Autodesk Inventor part; units mm, degrees
ref_plane "YZ Plane" through (0, 0, 0) normal (1, 0, 0) x (0, 1, 0)
ref_plane "XZ Plane" through (0, 0, 0) normal (0, 1, 0) x (-1, 0, 0)
ref_plane "XY Plane" through (0, 0, 0) normal (0, 0, 1) x (1, 0, 0)
sketch "Sketch1" plane through (0, 0, 0) normal (0, 0, 1) x (1, 0, 0)
  line L0 (-35.3228, 16.049) -> (-9.9228, 16.049)
  line L1 (-9.9228, 16.049) -> (-9.9228, -34.751)
  line L2 (-9.9228, -34.751) -> (-35.3228, -34.751)
  line L3 (-35.3228, -34.751) -> (-35.3228, 16.049)
  line L4 (-13.0978, 12.874) -> (-32.1478, 12.874)
  line L5 (-32.1478, 12.874) -> (-32.1478, -31.576)
  line L6 (-32.1478, -31.576) -> (-13.0978, -31.576)
  line L7 (-13.0978, -31.576) -> (-13.0978, 12.874)
  point P0 (0, 0)
  dimension "d0" = 25.4
  dimension "d1" = 50.8
  dimension "d2" = 3.175
extrude "Extrusion1" add sketch "Sketch1" along normal blind 977.9
sketch "Sketch2" plane through (-35.3228, -34.751, 0) normal (-1, 0, 0) x (0, 0, 1)
  line L0 (0, 0) -> (0, 50.8) construction
  line L1 (0, 25.4) -> (25.4, 25.4) construction
  circle A0 centre (25.4, 25.4) radius 12.7
  point P0 (0, 34.751)
  dimension "d5" = 25.4
  dimension "d9" = 25.4
extrude "Extrusion2" cut sketch "Sketch2" against normal blind 12.7
sketch "Sketch3" plane through (-35.3228, -34.751, 0) normal (-1, 0, 0) x (0, 0, 1)
  line L0 (977.9, 50.8) -> (977.9, 0) construction
  line L1 (977.9, 25.4) -> (800.1, 25.4) construction
  circle A0 centre (800.1, 25.4) radius 14.2875
  point P0 (0, 34.751)
  dimension "d10" = 177.8
  dimension "d11" = 28.575
extrude "Extrusion3" cut sketch "Sketch3" against normal blind 25.4
sketch "Sketch4" plane through (-35.3228, -34.751, 0) normal (-1, 0, 0) x (0, 0, 1)
  line L0 (977.9, 50.8) -> (977.9, 0) construction
  line L1 (977.9, 25.4) -> (419.1, 25.4) construction
  circle A0 centre (419.1, 25.4) radius 14.2875
  point P0 (0, 34.751)
  dimension "d14" = 558.8
  dimension "d15" = 28.575
extrude "Extrusion4" cut sketch "Sketch4" against normal blind 25.4
sketch "Sketch5" plane through (-35.3228, -34.751, 0) normal (-1, 0, 0) x (0, 0, 1)
  circle A0 centre (419.1, 25.4) radius 14.2875 construction
  line L0 (419.1, 25.4) -> (401.1395, 7.4395) construction
  line L1 (419.1, 25.4) -> (444.5, 25.4) construction
  line L2 (419.1, 25.4) -> (437.0605, 43.3605) construction
  circle A1 centre (401.1395, 7.4395) radius 2.032
  circle A2 centre (437.0605, 43.3605) radius 2.032
  point P0 (0, 34.751)
  dimension "d18" = 25.4
  dimension "d19" = 135
  dimension "d20" = 25.4
  dimension "d21" = 4.064
  dimension "d22" = 4.064
extrude "Extrusion5" cut sketch "Sketch5" against normal blind 25.4
sketch "Sketch7" plane through (-9.9228, -34.751, 0) normal (1, 0, 0) x (0, 0, -1)
  line L0 (0, 0) -> (0, 50.8) construction
  line L1 (0, 25.4) -> (-25.4, 25.4) construction
  circle A0 centre (-25.4, 25.4) radius 14.2875
  point P0 (0, 34.751)
  dimension "d34" = 25.4
  dimension "d35" = 28.575
extrude "Extrusion7" cut sketch "Sketch7" against normal blind 12.7
sketch "Sketch8" plane through (-9.9228, -34.751, 0) normal (1, 0, 0) x (0, 0, -1)
  circle A0 centre (-25.4, 25.4) radius 14.2875 construction
  line L0 (-25.4, 25.4) -> (-25.4, 49.2125) construction
  line L1 (-25.4, 49.2125) -> (-4.7778, 37.3063) construction
  line L2 (-4.7778, 37.3063) -> (-4.7778, 13.4938) construction
  line L3 (-4.7778, 13.4938) -> (-25.4, 1.5875) construction
  line L4 (-25.4, 1.5875) -> (-46.0222, 13.4937) construction
  line L5 (-46.0222, 13.4937) -> (-46.0222, 37.3062) construction
  line L6 (-46.0222, 37.3062) -> (-25.4, 49.2125) construction
  circle A1 centre (-4.7778, 37.3063) radius 2.5797
  circle A2 centre (-4.7778, 13.4938) radius 2.5797
  circle A3 centre (-46.0222, 13.4937) radius 2.5797
  circle A4 centre (-46.0222, 37.3062) radius 2.5797
  point P0 (0, 34.751)
  dimension "d45" = 23.8125
  dimension "d46" = 5.1594
  dimension "d47" = 5.1594
  dimension "d48" = 5.1594
  dimension "d49" = 5.1594
extrude "Extrusion9" cut sketch "Sketch8" against normal blind 25.4
sketch "Sketch9" plane through (0, 0, 0) normal (0, 0, -1) x (-1, 0, 0)
  line L0 (9.9228, 16.049) -> (35.3228, 16.049)
  line L1 (9.9228, 16.049) -> (13.0978, 16.049)
  line L2 (13.0978, 16.049) -> (13.0978, -34.751)
  line L3 (13.0978, -34.751) -> (9.9228, -34.751)
  line L4 (9.9228, -34.751) -> (9.9228, 16.049)
  line L5 (9.9228, -34.751) -> (35.3228, -34.751)
  line L6 (35.3228, -34.751) -> (35.3228, -31.576)
  line L7 (35.3228, -31.576) -> (9.9228, -31.576)
  line L8 (9.9228, -31.576) -> (9.9228, -34.751)
  line L9 (9.9228, -34.751) -> (35.3228, -34.751)
  line L10 (35.3228, -34.751) -> (32.1478, -34.751)
  line L11 (32.1478, -34.751) -> (32.1478, 16.049)
  line L12 (32.1478, 16.049) -> (35.3228, 16.049)
  line L13 (35.3228, 16.049) -> (35.3228, -34.751)
  line L14 (35.3228, 16.049) -> (9.9228, 16.049)
  line L15 (9.9228, 16.049) -> (9.9228, 12.874)
  line L16 (9.9228, 12.874) -> (35.3228, 12.874)
  line L17 (35.3228, 12.874) -> (35.3228, 16.049)
  point P0 (0, 0)
  dimension "d52" = 3.175
  dimension "d53" = 50.8
  dimension "d54" = 25.4
  dimension "d55" = 3.175
  dimension "d56" = 3.175
  dimension "d57" = 50.8
  dimension "d58" = 25.4
  dimension "d59" = 3.175
extrude "Extrusion10" add sketch "Sketch9" along normal blind 12.7 contours L0 L2 L16 L4 | L0 L11 L16 L2 | L16 L2 L7 L4 | L0 L13 L16 L11 | L7 L2 L3 L4 | L16 L13 L7 L11 | L7 L11 L5 L2 | L7 L6 L5 L11
sketch "Sketch10" plane through (-35.3228, 16.049, 977.9) normal (0, 1, 0) x (1, 0, 0)
  line L0 (3.175, 0) -> (22.225, 0) construction
  line L1 (12.7, 0) -> (12.7, 508) construction
  line L2 (12.7, 0) -> (520.7, 0) construction
  circle A0 centre (12.7, 508) radius 2.5797
  point P0 (35.3228, 977.9)
  dimension "d62" = 508
  dimension "d63" = 90
  dimension "d64" = 5.1594
extrude "Extrusion11" cut sketch "Sketch10" against normal blind 101.6
properties part number "41.75in Arm Beam Alternate (Right)"
Geometry: final body of the model. Coordinates: model frame, mm. A direction names the side the tool comes from. Round coordinates to 2 decimals unless told otherwise and drop trailing zeros. Loops run counter-clockwise (first coordinate to the right, second up) from the corner with the lowest first, then second, coordinate; pieces in that order, holes last.
Q1. Section A-A on z = 419.1. Return loops of the section in (x, y), plus the area to 3 significant figures.
Q2. Access query for faces 5 (the flat face through (-23, -31.576, 476)), 6 (the cylindrical face through (-11.5, -23.3, 28.5)), 7 (the cylindrical face through (-11.53, -14.82, 432.3)). Directions: +Z, -Z, +X, -X, +Y, -Y. A direction counts if a zero-diameter tool reaches every point of the face in a straight line with its end or side. Return the directions, or none.
Q3. Pull-direction query (X, two-part tool) for faces 1 (the flat face through (-32.148, -9, 476)), 2 (the flat face through (-23, 16.049, 476)), 3 (the flat face through (-22, 12.874, 476)), 4 (the flat face through (-9.923, -9, 476)); classes: released by +X, released by -X, zero draft, split by the parting line, or undercut.
Q4. Material intervals for L1, parallel to Y at x = -28.25, z = 840.5; L2, parallel to X at y = -32, z = 469; L3, parallel to X at y = -27.5, z = 97, sorted ascending.
Q5. Pin query (flat end, axial travel): P1, Ø4.5, axis at y = -21.26, z = 46.02, coming from the -X side; P2, Ø6.5, axis at y = -21.26, z = 46.02, coming from the +X side. Return the tip coordinate at first contact, or that it passes through.
Q6. Section B-B on z = 889.5. Return loops of the section in (x, y), plus the area to 3 significant figures.
Q7. Section C-C on z = 25.4. Return loops of the section in (x, y), plus the area to 3 significant figures.
Evaluation:
1. outline: (-35.32, -34.75) - (-9.92, -34.75) - (-9.92, -23.64) - (-13.1, -23.64) - (-13.1, -31.58) - (-32.15, -31.58) - (-32.15, -23.64) - (-35.32, -23.64) - close; (-35.32, 4.94) - (-32.15, 4.94) - (-32.15, 12.87) - (-13.1, 12.87) - (-13.1, 4.94) - (-9.92, 4.94) - (-9.92, 16.05) - (-35.32, 16.05) - close
1. area: 262 mm2
2. face 5: +Z, -Z
2. face 6: +X
2. face 7: +X, -X
3. face 1: undercut
3. face 2: zero draft
3. face 3: undercut
3. face 4: released by +X
4. L1: y = -34.75 to -31.58, 12.87 to 16.05
4. L2: x = -35.32 to -25.04, -20.21 to -9.92
4. L3: x = -35.32 to -32.15, -13.1 to -9.92
5. P1: passes through
5. P2: stops at x = -9.92
6. outline: (-35.32, -34.75) - (-9.92, -34.75) - (-9.92, 16.05) - (-35.32, 16.05) - close; hole (-32.15, -31.58) - (-13.1, -31.58) - (-13.1, 12.87) - (-32.15, 12.87) - close
6. area: 444 mm2
7. outline: (-35.32, -34.75) - (-9.92, -34.75) - (-9.92, -23.64) - (-13.1, -23.64) - (-13.1, -31.58) - (-32.15, -31.58) - (-32.15, -22.05) - (-35.32, -22.05) - close; (-35.32, 3.35) - (-32.15, 3.35) - (-32.15, 12.87) - (-13.1, 12.87) - (-13.1, 4.94) - (-9.92, 4.94) - (-9.92, 16.05) - (-35.32, 16.05) - close
7. area: 272 mm2
